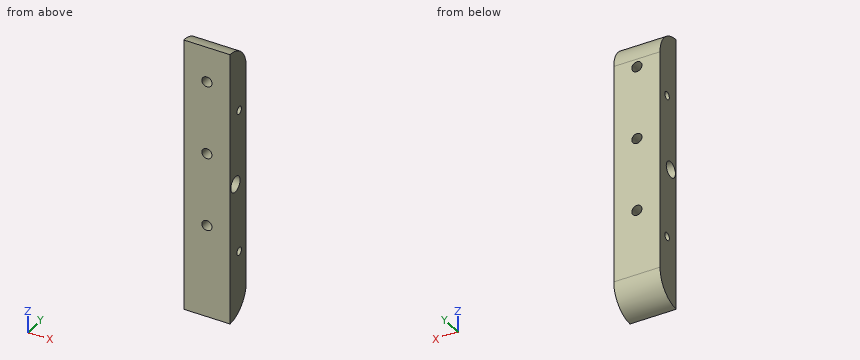
Autodesk Inventor part; units mm, degrees
ref_plane "YZ Plane" through (0, 0, 0) normal (1, 0, 0) x (0, 1, 0)
ref_plane "XZ Plane" through (0, 0, 0) normal (0, 1, 0) x (-1, 0, 0)
ref_plane "XY Plane" through (0, 0, 0) normal (0, 0, 1) x (1, 0, 0)
sketch "Sketch1" plane through (0, 0, 0) normal (1, 0, 0) x (0, 1, 0)
  line L0 (-7.5, 75) -> (7.5, 75)
  line L1 (7.5, 75) -> (7.5, -75)
  line L2 (7.5, -75) -> (-7.5, -75)
  line L3 (-7.5, -75) -> (-7.5, 75)
  line L4 (-7.5, 75) -> (7.5, -75) construction
  line L5 (7.5, 75) -> (-7.5, -75) construction
  point P0 (0, 0)
  dimension "d0" = 15
  dimension "d1" = 150
extrude "Extrusion1" add sketch "Sketch1" along normal blind 25
sketch "Sketch2" plane through (25, 0, 0) normal (1, 0, 0) x (0, 0, -1)
  circle A0 centre (-39.23, 1) radius 2.1
  circle A1 centre (39.23, 1) radius 2.1
  line L0 (-75, -7.5) -> (75, -7.5)
  line L1 (-75, 7.5) -> (-75, -7.5)
  line L2 (75, -7.5) -> (75, 7.5)
  point P0 (0, 0)
  dimension "d4" = 4.2
  dimension "d5" = 4.2
  dimension "d6" = 8.5
  dimension "d7" = 78.46
  dimension "d8" = 35.77
  dimension "d9" = 8.5
  dimension "d10" = 35.77
extrude "Extrusion2" cut sketch "Sketch2" against normal blind 25
fillet "Fillet1" radius 15 2 edges at (12.5, 7.5, 75) (12.5, 7.5, -75)
sketch "Sketch3" plane through (25, 0, 0) normal (1, 0, 0) x (0, 0, -1)
  circle A0 centre (0, -2.5) radius 4.25
  line L0 (60, 7.5) -> (-60, 7.5)
  arc A1 (75, -7.5) -> (60, 7.5) centre (60, -7.5) ccw
  point P0 (0, 0)
  dimension "d14" = 8.5
  dimension "d15" = 10
  dimension "d16" = 60
extrude "Extrusion3" cut sketch "Sketch3" against normal blind 25
sketch "Sketch4" plane through (0, 7.5, 60) normal (0, 1, 0) x (1, 0, 0)
  circle A0 centre (12.5, 4.23) radius 2.75
  circle A1 centre (12.5, 44.23) radius 2.75
  circle A2 centre (12.5, 84.23) radius 2.75
  point P0 (0, 60)
extrude "Extrusion4" cut sketch "Sketch4" against normal blind 25
properties part number "Plastic Holders" material "PC/ABS Plastic"
Read the model definition and answer for the solid it produces. Units are mm, in the model's axes. Round coordinates to 2 decimals unless told otherwise and drop trailing zeros. Order: outer loops, then holes, each group sorted by start corner. A loop starts at its lowest first (then second) coordinate and runs counter-clockwise, first axis right, second up. Notation, with made-up numbers: (-21.5, -4) - (31.5, -4) arc R27 ccw to (31.5, 14) - close; hole circle Ø11 at (44, -3). An arc over 180 degrees is marked (long way). Use one line per item in the form item = value. Start each with the question number.
(1) The part is cut by section D-D (z = 0). Give the vertices of the cut face in (x, y), then the cut area to 4 significant figures.
(2) The part is cut by section B-B (x = 8). Count the separate pieces of the cut face and the enclosed holes in it, then the cut area to 3 significant figures.
(3) The part is cut by section A-A (z = 39.23). Give the vertices of the cut face in (x, y).
(4) The part is cut by section C-C (y = -2.5). Give the vertices of the cut face in (x, z), then the cut area to 3 significant figures.
(5) Flat-ended cylindrical pins translate along their axes: pin 1 Ø3 at (x, y) = (3.5, -2.5) entering from -Z; pin 2 Ø1 at (x, y) = (4, -3.5) entering from +Z. Find the tip coordinate at first contact, or state that the pin passes through.
(6) Find the intervals of material crossed by line 1 along Y through (x, z) = (8, 39.23); line 2 along Z through (x, y) = (12.5, -3.75); line 3 along Z through (x, y) = (12.5, -4.5), in increasing order. Write a range as from..to.
Checked values:
q1.outline = (0, -7.5) - (25, -7.5) - (25, -6.75) - (0, -6.75) - close; (0, 1.75) - (25, 1.75) - (25, 7.5) - (0, 7.5) - close
q1.area = 162.5 mm^2
q2.separate_pieces = 1
q2.enclosed_holes = 3
q2.area = 2,070 mm^2
q3.outline = (0, -7.5) - (25, -7.5) - (25, -1.1) - (0, -1.1) - close; (0, 3.1) - (25, 3.1) - (25, 7.5) - (0, 7.5) - close
q4.outline = (0, -74.14) - (25, -74.14) - (25, -4.25) - (0, -4.25) - close; (0, 4.25) - (25, 4.25) - (25, 74.14) - (0, 74.14) - close; hole circle Ø5.5 at (12.5, -24.23); hole circle Ø5.5 at (12.5, 15.77); hole circle Ø5.5 at (12.5, 55.77)
q4.area = 3,420 mm^2
q5.pin_1 = -74.59
q5.pin_2 = 74.59
q6.line_1 = -7.5..-1.1, 3.1..7.5
q6.line_2 = -74.52..-26.98, -21.48..-4.06, 4.06..13.02, 18.52..53.02, 58.52..74.52
q6.line_3 = -74.7..-26.98, -21.48..-3.75, 3.75..13.02, 18.52..53.02, 58.52..74.7
